The model under review builds one solid part; all positions refer to its coordinate system, in mm. Round coordinates to 2 decimals unless told otherwise and drop trailing zeros. Order: outer loops, then holes, each group sorted by start corner. A loop starts at its lowest first (then second) coordinate and runs counter-clockwise, first axis right, second up. Notation, with made-up numbers: (-38.75, 22.5) -> (13.25, 22.5) arc R13 cw to (13.25, 31.5) -> close; hole circle Ø3 at (18.5, 53). An arc over 180 degrees is marked (long way). Use a Markdown table: item, result. Add a question column.
```python
from build123d import *

# Parameters (mm, degrees)
SKETCH1_R           = 4.445
BOSS_EXTRUDE1_DEPTH = 3.175
BOSS_EXTRUDE2_DEPTH = 1.27


with BuildPart() as part:
    # Sketch1 → Boss-Extrude1 (new body)
    with BuildSketch(Plane(origin=(0, 0, 0), x_dir=(1, 0, 0), z_dir=(0, 1, 0))):
        with Locations(Location((0, 0, 0), (0, 0, 270))):
            Circle(SKETCH1_R)
    extrude(amount=BOSS_EXTRUDE1_DEPTH)

    # Sketch3 → Boss-Extrude2 (add)
    with BuildSketch(Plane.XZ):
        with BuildLine():
            Line((0, 4.445), (0, 5.08))
            Line((0, 5.08), (-1.016, 5.08))
            Line((-1.016, 5.08), (-1.016, 4.327328159))
            ThreePointArc((-1.016, 4.327328159), (-0.511395801, 4.415484043), (0, 4.445))
        make_face()
        with BuildLine():
            Line((1.016, 4.327328159), (1.016, 5.08))
            Line((1.016, 5.08), (0, 5.08))
            Line((0, 5.08), (0, 4.445))
            ThreePointArc((0, 4.445), (0.511395801, 4.415484043), (1.016, 4.327328159))
        make_face()
    extrude(amount=-BOSS_EXTRUDE2_DEPTH)


solid = part.part
```
Q1. Add section D-D, the plane x = 3.5. Give the boundary of the cut face in (y, z) (3 decimals), then the cut area to 3 significant figures.
Q2. Draft analysis for pull direction Y (two halves, no side actions). For faces 1 (the face through (0, 0, 0)), 2 (the face through (0, 1, 5.08)), 3 (the face through (0, 3.175, 0)), state which applies: released by +Y, released by -Y, zero draft, split by the parting line, or undercut.
Q3. Add section C-C, the plane y = 1. Give the boundary of the cut face in (x, z) (3 decimals).
Q4. Add section B-B, the plane y = 2.5. Give the boundary of the cut face in (x, z) (3 decimals).
Q5. To check wall thickness, follow line 1 along Z through (x, y) = (-2.5, 1.5); line 2 along Z through (x, y) = (-3.5, 0.55); line 3 along X through (y, z) = (0.85, 1.75). State the ranges of each line that lie inside material, in increasing order.
Q6. For pin 1 (0.8 mm diameter, centred on y = 1, z = 4.5, fed in from -X), flat-tipped, find the tip position at first contact; note if it passes through.
Q7. Add section A-A, the plane x = 0. Give the boundary of the cut face in (y, z) (3 decimals), then the cut area to 3 significant figures.
Return value:
| question | item | result |
|---|---|---|
| 1 | outline | (0, -2.74) -> (3.175, -2.74) -> (3.175, 2.74) -> (0, 2.74) -> close |
| 1 | area | 17.4 mm² |
| 2 | face 1 | released by -Y |
| 2 | face 2 | zero draft |
| 2 | face 3 | released by +Y |
| 3 | outline | (-1.016, 4.327) arc R4.445 ccw (long way) to (1.016, 4.327) -> (1.016, 5.08) -> (-1.016, 5.08) -> close |
| 4 | outline | circle Ø8.89 at (0, 0) |
| 5 | line 1 | -3.68 to 3.68 |
| 5 | line 2 | -2.74 to 2.74 |
| 5 | line 3 | -4.09 to 4.09 |
| 6 | pin 1 | x = -1.72 |
| 7 | outline | (0, -4.445) -> (3.175, -4.445) -> (3.175, 4.445) -> (1.27, 4.445) -> (1.27, 5.08) -> (0, 5.08) -> close |
| 7 | area | 29.0 mm² |
